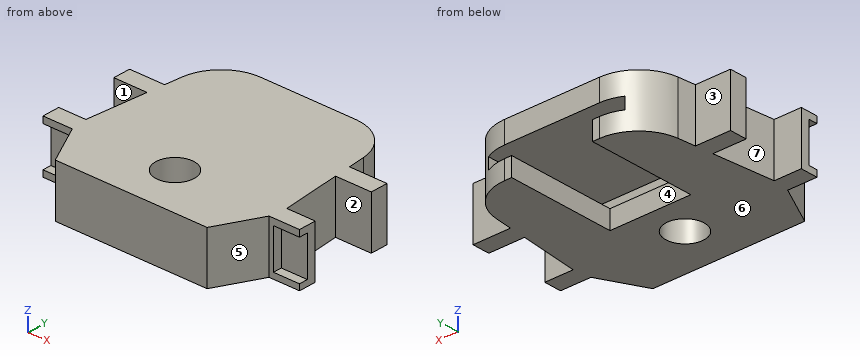
from build123d import *

# Parameters (mm, degrees)
SKETCH2_R           = 4.4
BOSS_EXTRUDE1_DEPTH = 12
CUT_EXTRUDE1_DEPTH  = 2
SKETCH4_W           = 31.5
SKETCH4_H           = 26.5
CUT_EXTRUDE2_DEPTH  = 2.7
CUT_EXTRUDE3_REACH  = 14
SKETCH5_W           = 18.640557444
SKETCH5_H           = 25


with BuildPart() as part:
    # Sketch2 → Boss-Extrude1 (new body)
    with BuildSketch(Plane.XY):
        with BuildLine():
            Line((-26.652708458, 24.799544054), (-27.052594325, 20.847218157))
            Line((-27.052594325, 20.847218157), (-35.117996865, 20.847218157))
            Line((-35.117996865, 20.847218157), (-35.117996865, 16.847218157))
            Line((-35.117996865, 16.847218157), (-27.457303732, 16.847218157))
            Line((-27.457303732, 16.847218157), (-28.873786654, 2.847218157))
            Line((-28.873786654, 2.847218157), (-35.117996865, 2.839337807))
            Line((-35.117996865, 2.839337807), (-35.112948764, -1.160662193))
            Line((-35.112948764, -1.160662193), (-28.37093921, -1.152153607))
            Line((-28.37093921, -1.152153607), (-23.24278353, -11.137592085))
            Line((-23.24278353, -11.137592085), (11.75721647, -11.137592085))
            Line((11.75721647, -11.137592085), (16.91451101, -1.09500223))
            Line((16.91451101, -1.09500223), (23.93161739, -1.086146466))
            Line((23.93161739, -1.086146466), (23.92656929, 2.913853534))
            Line((23.92656929, 2.913853534), (17.382313229, 2.905594519))
            Line((17.382313229, 2.905594519), (15.971736672, 16.847218157))
            Line((15.971736672, 16.847218157), (24.207665477, 16.847218157))
            Line((24.207665477, 16.847218157), (24.207665477, 20.847218157))
            Line((24.207665477, 20.847218157), (15.567027266, 20.847218157))
            Line((15.567027266, 20.847218157), (15.167141399, 24.799544054))
            ThreePointArc((15.167141399, 24.799544054), (11.923667067, 31.21134436), (5.217936029, 33.792909804))
            Line((5.217936029, 33.792909804), (-16.703503089, 33.792909804))
            ThreePointArc((-16.703503089, 33.792909804), (-23.409234126, 31.21134436), (-26.652708458, 24.799544054))
        make_face()
        with Locations((-5.74278353, 0)):
            Circle(SKETCH2_R, mode=Mode.SUBTRACT)
    extrude(amount=BOSS_EXTRUDE1_DEPTH)

    # Sketch3 → Cut-Extrude1 (cut)
    with BuildSketch(Plane(origin=(0.001408858, -1.116346991, 0), x_dir=(0.999999204, 0.001262024, 0), z_dir=(0.001262024, -0.999999204, 0))):
        Polygon((-35.114385586, 10.5), (-29.114385586, 10.5), (-29.114385586, 8.5), (-29.114385586, 3.523848556), (-29.114385586, 1.461924081), (-35.114385586, 1.461924081), (-35.114385586, 3.523848556), (-35.114385586, 8.5), align=None)
        Polygon((17.930227589, 10.5), (23.930227589, 10.5), (23.930227589, 8.5), (23.930227589, 3.438075525), (23.930227589, 1.376151049), (17.930227589, 1.376151049), (17.930227589, 3.438075525), (17.930227589, 8.5), align=None)
    extrude(amount=-CUT_EXTRUDE1_DEPTH, mode=Mode.SUBTRACT)

    # Sketch4 → Cut-Extrude2 (cut)
    with BuildSketch(Plane.XY.offset(7)):
        with Locations((-5.74278353, 20.542909804)):
            Rectangle(SKETCH4_W, SKETCH4_H)
    extrude(amount=-CUT_EXTRUDE2_DEPTH, mode=Mode.SUBTRACT)

    # Sketch5 → Cut-Extrude3 (cut, up to next)
    with BuildSketch(Plane(origin=(0, 0, 0), x_dir=(-1, 0, 0), z_dir=(0, 0, -1)), mode=Mode.PRIVATE) as cut_extrude3_sk1:
        with Locations((5.74278353, 21.292909804)):
            Rectangle(SKETCH5_W, SKETCH5_H)
    cut_extrude3_tool1 = extrude(cut_extrude3_sk1.sketch, amount=-CUT_EXTRUDE3_REACH, mode=Mode.PRIVATE) & part.part
    add(cut_extrude3_tool1.solids().sort_by_distance((-5.742784, 21.29291, 0))[0], mode=Mode.SUBTRACT)


solid = part.part
Input: part model. Units: mm. Frame: model coordinates. Face numbers are marked on the shaded views. A direction names the side the tool comes from. Coordinates: 2 decimals unless noted, no trailing zeros. Order: outer loops, then holes, each group sorted by start corner. A loop starts at its lowest first (then second) coordinate and runs counter-clockwise, first axis right, second up.
1. Draft query along Y for the marked faces 4, 5, 6 and 7. Return one class per face: +Y half, -Y half, draft (parallel to the pull), parting line (faces both ways), or undercut.
Checked values:
face 4: +Y half
face 5: -Y half
face 6: draft
face 7: undercut
2. Cut plane D-D, the plane y = 12. Return loops of the section in (x, z).
Checked values:
outline: (-27.95, 0) - (-15.06, 0) - (-15.06, 4.3) - (-21.49, 4.3) - (-21.49, 7) - (10.01, 7) - (10.01, 4.3) - (3.58, 4.3) - (3.58, 0) - (16.46, 0) - (16.46, 12) - (-27.95, 12) - close
3. Contact query for flat-ended pins moving along their axis: P1, Ø6.5, axis at x = 22, z = 8, coming from the -Y side; P2, Ø1.4, axis at y = 24, z = 5, coming from the -X side; P3, Ø2, axis at y = 22.5, z = 6, coming from the +X side; P4, Ø10, axis at x = -28.5, y = 4.5, coming from the -Z side. Output: stop coordinate, or through.
Checked values:
P1: stops at y = -1.09
P2: stops at x = -26.8
P3: stops at x = 15.5
P4: stops at z = 0
4. Ray query, line 1 along Y through (x, z) = (20.5, 11); line 2 along X through (y, z) = (20, 1.75); line 3 along X through (y, z) = (3, 2.25). Return the intervals inside material, ascending.
Checked values:
line 1: y = -1.09 to 2.91, 16.85 to 20.85
line 2: x = -35.12 to -15.06, 3.58 to 24.21
line 3: x = -28.86 to -8.96, -2.52 to 17.37
5. Cut plane C-C, the plane y = 20. Return loops of the section in (x, z).
Checked values:
outline: (-35.12, 0) - (-15.06, 0) - (-15.06, 4.3) - (-21.49, 4.3) - (-21.49, 7) - (10.01, 7) - (10.01, 4.3) - (3.58, 4.3) - (3.58, 0) - (24.21, 0) - (24.21, 12) - (-35.12, 12) - close
6. Cut plane B-B, the plane x = 0. Return loops of the section in (y, z), plus the area to 3 significant figures.
Checked values:
outline: (-11.14, 0) - (8.79, 0) - (8.79, 4.3) - (7.29, 4.3) - (7.29, 7) - (33.79, 7) - (33.79, 12) - (-11.14, 12) - close
area: 360 mm2
7. Access query for the marked faces 1, 2 and 3. Directions: +Z, -Z, +X, -X, +Y, -Y. A direction counts if a zero-diameter tool reaches every point of the face in a straight line with its end or side. Return the directions, or none.
Checked values:
face 1: +Z, -Z, -X
face 2: +Z, -Z, +X
face 3: +Z, -Z, -X, +Y
8. Cut plane A-A, the plane y = 0. Return loops of the section in (x, z), plus the area to 3 significant figures.
Checked values:
outline: (-35.11, 0) - (-10.14, 0) - (-10.14, 12) - (-35.11, 12) - (-35.11, 10.5) - (-29.11, 10.5) - (-29.11, 1.46) - (-35.11, 1.46) - close; (-1.34, 0) - (23.93, 0) - (23.93, 1.38) - (17.93, 1.38) - (17.93, 10.5) - (23.93, 10.5) - (23.93, 12) - (-1.34, 12) - close
area: 494 mm2
